```python
from build123d import *

# Parameters (mm, degrees)
SKETCH1_R           = 2.5
BOSS_EXTRUDE1_DEPTH = 225
FILLET1_R           = 1.065
FILLET2_R           = 2.13


with BuildPart() as part:
    # Sketch1 → Boss-Extrude1 (new body)
    with BuildSketch(Plane.YZ):
        Polygon((-12.5, -3.25), (-12.5, -12.5), (-3.25, -12.5), (-3.25, -10.37), (-8.863862556, -10.37), (-2.873862556, -4.38), (2.873862556, -4.38), (8.863862556, -10.37), (3.25, -10.37), (3.25, -12.5), (12.5, -12.5), (12.5, -3.25), (10.37, -3.25), (10.37, -8.863862556), (4.38, -2.873862556), (4.38, 2.873862556), (10.37, 8.863862556), (10.37, 3.25), (12.5, 3.25), (12.5, 12.5), (3.25, 12.5), (3.25, 10.37), (8.863862556, 10.37), (2.873862556, 4.38), (-2.873862556, 4.38), (-8.863862556, 10.37), (-3.25, 10.37), (-3.25, 12.5), (-12.5, 12.5), (-12.5, 3.25), (-10.37, 3.25), (-10.37, 8.863862556), (-4.38, 2.873862556), (-4.38, -2.873862556), (-10.37, -8.863862556), (-10.37, -3.25), align=None)
        with Locations(Location((0, 0, 0), (0, 0, 270))):
            Circle(SKETCH1_R, mode=Mode.SUBTRACT)
    extrude(amount=BOSS_EXTRUDE1_DEPTH)

    # Fillet1
    fillet1_edges = [part.edges().sort_by_distance(p)[0] for p in [
        (112.5, -10.37, -8.863862556),
        (112.5, 2.873862556, -4.38),
        (112.5, -2.873862556, -4.38),
        (112.5, -4.38, 2.873862556),
        (112.5, -4.38, -2.873862556),
        (112.5, -2.873862556, 4.38),
        (112.5, 2.873862556, 4.38),
        (112.5, 4.38, 2.873862556),
        (112.5, 4.38, -2.873862556),
        (112.5, -8.863862556, -10.37),
        (112.5, 8.863862556, -10.37),
        (112.5, 10.37, -8.863862556),
        (112.5, -10.37, 8.863862556),
        (112.5, -8.863862556, 10.37),
        (112.5, 10.37, 8.863862556),
        (112.5, 8.863862556, 10.37),
        (112.5, 12.5, 3.25),
        (112.5, -3.25, -12.5),
        (112.5, -10.37, 3.25),
        (112.5, 10.37, 3.25),
        (112.5, -10.37, -3.25),
        (112.5, -12.5, -3.25),
        (112.5, -12.5, 3.25),
        (112.5, 3.25, -10.37),
        (112.5, -3.25, -10.37),
        (112.5, 3.25, -12.5),
        (112.5, 10.37, -3.25),
        (112.5, 12.5, -3.25),
        (112.5, 3.25, 12.5),
        (112.5, 3.25, 10.37),
        (112.5, -3.25, 10.37),
        (112.5, -3.25, 12.5),
    ]]
    fillet(fillet1_edges, radius=FILLET1_R - 0.0001)  # a hair under: the kernel refuses the full size

    # Fillet2
    fillet2_edges = [part.edges().sort_by_distance(p)[0] for p in [
        (112.5, -12.5, 12.5),
        (112.5, 12.5, 12.5),
        (112.5, 12.5, -12.5),
        (112.5, -12.5, -12.5),
    ]]
    fillet(fillet2_edges, radius=FILLET2_R)


solid = part.part
```
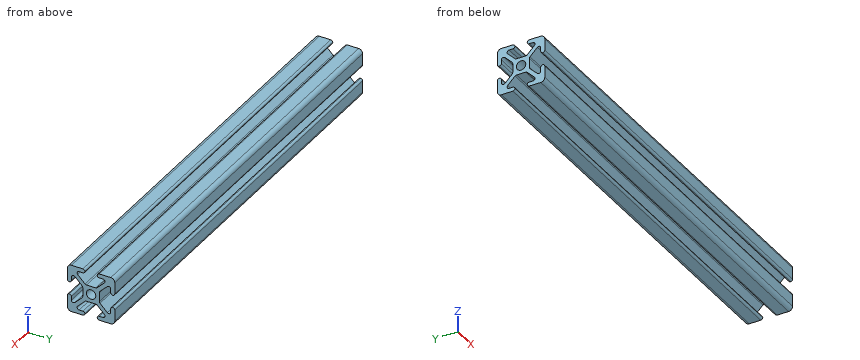
Read the model definition and answer for the solid it produces. Units are mm, in the model's axes. Coordinates: 2 decimals unless noted, no trailing zeros. Write each loop counter-clockwise with the first axis right and the second up, starting at its lowest first coordinate (ties: lowest second). Pieces come first, ordered by that corner, then holes. Notation, with made-up numbers: (-35.75, 1.5) -> (-9.75, 1.5) arc R22 ccw to (-9.75, 29.5) -> close; hole circle Ø9 at (72, -5.75). An arc over 180 degrees is marked (long way). Return JSON: item names as keys, results as strings.
1. A cutting plane is placed at A-A (y = 0). Determine the outline of the cut face in (x, z), and give its area (3 significant figures).
Found:
{"outline": "(0, -4.38) -> (225, -4.38) -> (225, -2.5) -> (0, -2.5) -> close; (0, 2.5) -> (225, 2.5) -> (225, 4.38) -> (0, 4.38) -> close", "area": "846 mm2"}
2. A cutting plane is placed at B-B (z = 0.5). Determine the outline of the cut face in (x, y).
Found:
{"outline": "(0, -4.38) -> (225, -4.38) -> (225, -2.45) -> (0, -2.45) -> close; (0, 2.45) -> (225, 2.45) -> (225, 4.38) -> (0, 4.38) -> close"}
3. Find the intervals of material crossed by line 1 along Z through (x, y) = (149.5, 9); line 2 along Y through (x, z) = (56, 0); line 3 along Z through (x, y) = (189, 4.5), in increasing order. Write a range as from..to.
Found:
{"line 1": "-12.5..-7.31, 7.31..12.5", "line 2": "-4.38..-2.5, 2.5..4.38", "line 3": "-12.5..-10.37, -6.01..-2.92, 2.92..6.01, 10.37..12.5"}
4. Each of these flat-tipped pins is pushed along its axis until it touches: P1, Ø2.5, axis at x = 84.5, z = 1, coming from the -Y side; P2, Ø4, axis at x = 87.5, z = 0, coming from the +Y side; P3, Ø4, axis at y = 1, z = 8.5, coming from the -X side; P4, Ø2.5, axis at x = 97.5, y = -1, coming from the -Z side. Where does it stop, or does it pass through?
Found:
{"P1": "y = -4.38", "P2": "y = 4.38", "P3": "through", "P4": "z = -4.38"}
